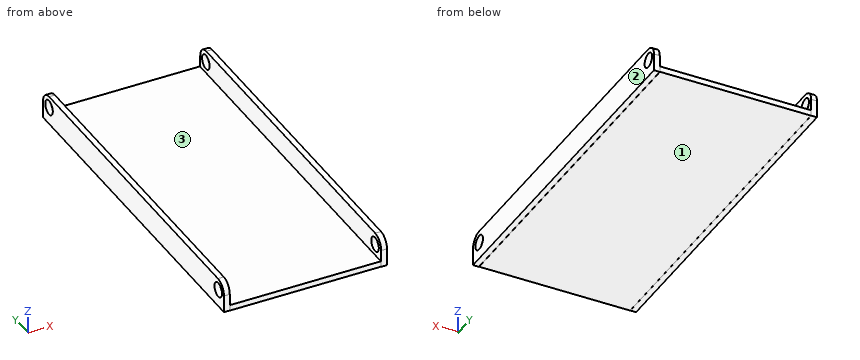
from build123d import *

# Parameters (mm, degrees)
F0_W     = 66.04
F0_H     = 152.4
F1_DEPTH = 2.54
F2_W     = 152.4
F2_H     = 12.7
F3_DEPTH = 2.54
F4_W     = 152.4
F4_H     = 12.7
F5_DEPTH = 2.54
F6_R     = 5.08
F7_R     = 3.175
F8_DEPTH = 90.17


with BuildPart() as f1:
    # F0 (on Top) → F1 (new body)
    with BuildSketch(Plane.XY):
        Rectangle(F0_W, F0_H)
    extrude(amount=F1_DEPTH)

    # F2 (on face) → F3 (join)
    with BuildSketch(Plane.YZ.offset(33.02)):
        with Locations((-0.243933, 6.454543)):
            Rectangle(F2_W, F2_H)
    extrude(amount=F3_DEPTH)

    # F4 (on face) → F5 (join)
    with BuildSketch(Plane(origin=(-33.02, 0, 0), x_dir=(0, -1, 0), z_dir=(-1, 0, 0))):
        with Locations((-0.127775, 6.291921)):
            Rectangle(F4_W, F4_H)
    extrude(amount=F5_DEPTH)

    # F6
    f6_edges = [f1.edges().sort_by_distance(p)[0] for p in [
        (34.29, -76.443933, 12.804543),
        (-34.29, -76.072225, 12.641921),
        (34.29, 75.956067, 12.804543),
        (-34.29, 76.327775, 12.641921),
    ]]
    fillet(f6_edges, radius=F6_R)

    # F7 (on face) → F8 (cut)
    with BuildSketch(Plane(origin=(-35.56, 0, 0), x_dir=(0, -1, 0), z_dir=(-1, 0, 0))):
        with Locations((-71.247775, 7.561921)):
            Circle(F7_R)
        with Locations((71.247775, 7.561921)):
            Circle(F7_R)
    extrude(amount=-F8_DEPTH, mode=Mode.SUBTRACT)


solid = f1.part
Input: part model. Units: mm. Frame: model coordinates. Face numbers are marked on the shaded views. Give positions to 0.01 mm unless a question says otherwise; leave off trailing zeros. Loops run counter-clockwise (first coordinate to the right, second up) from the corner with the lowest first, then second, coordinate; pieces in that order, holes last. Notation, with made-up numbers: (49, 86) -> (70, 86) arc R19 ccw to (70, 90) -> close; hole circle Ø11 at (10, -27). An arc over 180 degrees is marked (long way). Answer as a JSON object with one key per item and string values. Group by question number.
Item 1: Pull-direction query (X, two-part tool) for the marked faces 1, 2 and 3; classes: released by +X, released by -X, zero draft, split by the parting line, or undercut.
Item 2: Cut plane B-B, the plane x = 9.5. Return the cut outline in (y, z), and give its area (3 significant figures).
Item 3: Cut plane A-A, the plane y = -8.5. Return the cut outline in (x, z).
Item 4: Pin query (flat end, axial travel): P1, Ø3, axis at x = 19, z = 1.5, coming from the -Y side; P2, Ø5, axis at x = 4, y = -39.5, coming from the +Z side; P3, Ø0.8, axis at x = 34.5, z = 5.5, coming from the +Y side; P4, Ø4, axis at y = 71.25, z = 7.56, coming from the +X side. Return the tip coordinate at first contact, or that it passes through.
Item 5: Line query: probe 1 along X at (y, z) = (48, 7.25); probe 2 along Z at (x, y) = (8.5, 66); probe 3 along Y at (x, z) = (-26.5, 1). Output: solid intervals per line, ascending.
Checks:
{
 "1": {"face 1": "zero draft", "face 2": "released by +X", "face 3": "undercut"},
 "2": {"outline": "(-76.2, 0) -> (76.2, 0) -> (76.2, 2.54) -> (-76.2, 2.54) -> close", "area": "387 mm²"},
 "3": {"outline": "(-35.56, -0.06) -> (-33.02, -0.06) -> (-33.02, 0) -> (33.02, 0) -> (33.02, 0.1) -> (35.56, 0.1) -> (35.56, 12.8) -> (33.02, 12.8) -> (33.02, 2.54) -> (-33.02, 2.54) -> (-33.02, 12.64) -> (-35.56, 12.64) -> close"},
 "4": {"P1": "stops at y = -76.2", "P2": "stops at z = 2.54", "P3": "stops at y = 75.96", "P4": "passes through"},
 "5": {"probe 1": "x = -35.56 to -33.02, 33.02 to 35.56", "probe 2": "z = 0 to 2.54", "probe 3": "y = -76.2 to 76.2"}
}
